Input: part model. Units: mm. Frame: model coordinates. A direction names the side the tool comes from. Coordinates: 2 decimals unless noted, no trailing zeros. Order: outer loops, then holes, each group sorted by start corner. A loop starts at its lowest first (then second) coordinate and runs counter-clockwise, first axis right, second up. Notation, with made-up numbers: M -34,19.25 L 11,19.25 A26 cw 11,38.25 Z; hole C 50,-21.75 d1. An arc over 180 degrees is marked long. One line per item, written item: value.
```python
from build123d import *

# Parameters (mm, degrees)
SKETCH1_R           = 2.5
BOSS_EXTRUDE1_DEPTH = 3.175


with BuildPart() as part:
    # Sketch1 → Boss-Extrude1 (new body)
    with BuildSketch(Plane(origin=(0, 0, 0), x_dir=(0, 0, -1), z_dir=(1, 0, 0))):
        Polygon((0, 0), (7.096461031, 0), (15.026461031, 7.93), (45.298538969, 7.93), (53.228538969, 0), (60.325, 0), (60.325, 22.86), (52.3875, 22.86), (52.3875, 26.035), (46.0375, 26.035), (46.0375, 22.86), (39.6875, 22.86), (39.6875, 26.035), (33.3375, 26.035), (33.3375, 22.86), (26.9875, 22.86), (26.9875, 26.035), (20.6375, 26.035), (20.6375, 22.86), (14.2875, 22.86), (14.2875, 26.035), (7.9375, 26.035), (7.9375, 22.86), (0, 22.86), align=None)
        with Locations((5.1625, 4.43)):
            Circle(SKETCH1_R, mode=Mode.SUBTRACT)
        with Locations(Location((55.1625, 4.43, 0), (0, 0, 180))):
            Circle(SKETCH1_R, mode=Mode.SUBTRACT)
    extrude(amount=BOSS_EXTRUDE1_DEPTH)


solid = part.part
```
(1) First-contact query: pin 1 (1 mm diameter, centred on x = 2, y = 25, fed in from -Z); pin 2 (1 mm diameter, centred on x = 0.5, z = -15.5, fed in from -Y); pin 3 (3 mm diameter, centred on y = 4.43, z = -55.16, fed in from +X); pin 4 (1.6 mm diameter, centred on x = 2, y = 24.5, fed in from +Z). Flat tips, straight axial feed; report the tip coordinate or a pass-through.
Data:
pin 1: stops at z = -52.39
pin 2: stops at y = 7.9
pin 3: passes through
pin 4: stops at z = -7.94
(2) Access query for faces 1 (the flat face through (2, 22.86, -4)), 2 (the flat face through (2, 24, -52.388)), 3 (the flat face through (2, 22.86, -30)). Directions: +Z, -Z, +X, -X, +Y, -Y. A direction counts if a zero-diameter tool reaches every point of the face in a straight line with its end or side. Return the directions, or none.
Data:
face 1: +Z, +X, -X, +Y
face 2: -Z, +X, -X, +Y
face 3: +X, -X, +Y
(3) Cut plane D-D on z = -49.5. Output: boundary loops of the cut face in (x, y) (3 decimals), plus the area to 3 significant figures.
Data:
outline: M 0,3.729 L 3.175,3.729 L 3.175,26.035 L 0,26.035 Z
area: 70.8 mm2
(4) Cut plane B-B on y = 4.43. Output: boundary loops of the cut face in (x, z) (1 decimal), plus the area to 3 significant figures.
Data:
outline: M 0,-60.3 L 3.2,-60.3 L 3.2,-57.7 L 0,-57.7 Z; M 0,-52.7 L 3.2,-52.7 L 3.2,-48.8 L 0,-48.8 Z; M 0,-11.5 L 3.2,-11.5 L 3.2,-7.7 L 0,-7.7 Z; M 0,-2.7 L 3.2,-2.7 L 3.2,0 L 0,0 Z
area: 41.4 mm2
(5) Cut plane A-A on x = 1.6. Output: boundary loops of the cut face in (y, z) (1 decimal), plus the area to 3 significant figures.
Data:
outline: M 0,-60.3 L 22.9,-60.3 L 22.9,-52.4 L 26,-52.4 L 26,-46 L 22.9,-46 L 22.9,-39.7 L 26,-39.7 L 26,-33.3 L 22.9,-33.3 L 22.9,-27 L 26,-27 L 26,-20.6 L 22.9,-20.6 L 22.9,-14.3 L 26,-14.3 L 26,-7.9 L 22.9,-7.9 L 22.9,0 L 0,0 L 0,-7.1 L 7.9,-15 L 7.9,-45.3 L 0,-53.2 Z; hole C 4.4,-55.2 d5; hole C 4.4,-5.2 d5
area: 1,120 mm2
(6) Draft query along Z for faces 4 (the flat face through (2, 24, -7.938)), 5 (the flat face through (1.565, 3.909, -11.006)), 6 (the flat face through (2, 0, -3)). Return one class per face: released by +Z, released by -Z, zero draft, split by the parting line, or undercut.
Data:
face 4: released by +Z
face 5: undercut
face 6: zero draft
(7) Cut plane C-C on z = -42. Output: boundary loops of the cut face in (x, y) (3 decimals), plus the area to 3 significant figures.
Data:
outline: M 0,7.93 L 3.175,7.93 L 3.175,22.86 L 0,22.86 Z
area: 47.4 mm2
(8) Ray query, line 1 (Y direction, x = 1.65, z = -55); line 2 (Y direction, x = 1.85, z = -39) (3 decimals); line 3 (Y direction, x = 0.3, z = -32). Return the intervals inside material, ascending. Write a range as from..to.
Data:
line 1: y = 0..1.94, 6.92..22.86
line 2: y = 7.93..26.035
line 3: y = 7.93..22.86
